```python
from build123d import *

# Parameters (mm, degrees)
SKETCH1_R           = 6.338085432
SKETCH1_W           = 63.5
SKETCH1_H           = 44.45
BOSS_EXTRUDE1_DEPTH = 2.54
BOSS_EXTRUDE2_DEPTH = 12.7
CUT_EXTRUDE1_REACH  = 136.65
SKETCH3_W           = 12.7
SKETCH3_H           = 12.7


with BuildPart() as part:
    # Sketch1 → Boss-Extrude1 (new body)
    with BuildSketch(Plane.XY):
        with BuildLine():
            Line((88.9, 99.06), (88.9, 2.54))
            ThreePointArc((88.9, 2.54), (88.156051224, 0.743948776), (86.36, 0))
            Line((86.36, 0), (2.54, 0))
            ThreePointArc((2.54, 0), (0.743948776, 0.743948776), (0, 2.54))
            Line((0, 2.54), (0, 99.06))
            ThreePointArc((0, 99.06), (0.743948776, 100.856051224), (2.54, 101.6))
            Line((2.54, 101.6), (86.36, 101.6))
            ThreePointArc((86.36, 101.6), (88.156051224, 100.856051224), (88.9, 99.06))
        make_face()
        with Locations((31.75, 25.352341726)):
            Circle(SKETCH1_R, mode=Mode.SUBTRACT)
        with Locations((44.366598021, 38.028512589)):
            Circle(SKETCH1_R, mode=Mode.SUBTRACT)
        with Locations((57.042768884, 25.352341726)):
            Circle(SKETCH1_R, mode=Mode.SUBTRACT)
        with Locations((44.366598021, 12.676170863)):
            Circle(SKETCH1_R, mode=Mode.SUBTRACT)
        with Locations((45.72, 75.565)):
            Rectangle(SKETCH1_W, SKETCH1_H, mode=Mode.SUBTRACT)
    extrude(amount=BOSS_EXTRUDE1_DEPTH)

    # Sketch2 → Boss-Extrude2 (add)
    with BuildSketch(Plane(origin=(0, 0, 0), x_dir=(-1, 0, 0), z_dir=(0, 0, -1))):
        with BuildLine():
            Line((-3.81, 100.33), (-85.09, 100.33))
            ThreePointArc((-85.09, 100.33), (-86.886051224, 99.586051224), (-87.63, 97.79))
            Line((-87.63, 97.79), (-87.63, 3.81))
            ThreePointArc((-87.63, 3.81), (-86.886051224, 2.013948776), (-85.09, 1.27))
            Line((-85.09, 1.27), (-3.81, 1.27))
            ThreePointArc((-3.81, 1.27), (-2.013948776, 2.013948776), (-1.27, 3.81))
            Line((-1.27, 3.81), (-1.27, 97.79))
            ThreePointArc((-1.27, 97.79), (-2.013948776, 99.586051224), (-3.81, 100.33))
        make_face()
        with BuildLine():
            ThreePointArc((-83.82, 99.06), (-85.616051224, 98.316051224), (-86.36, 96.52))
            Line((-86.36, 96.52), (-86.36, 5.08))
            ThreePointArc((-86.36, 5.08), (-85.616051224, 3.283948776), (-83.82, 2.54))
            Line((-83.82, 2.54), (-5.08, 2.54))
            ThreePointArc((-5.08, 2.54), (-3.283948776, 3.283948776), (-2.54, 5.08))
            Line((-2.54, 5.08), (-2.54, 96.52))
            ThreePointArc((-2.54, 96.52), (-3.283948776, 98.316051224), (-5.08, 99.06))
            Line((-5.08, 99.06), (-83.82, 99.06))
        make_face(mode=Mode.SUBTRACT)
    extrude(amount=BOSS_EXTRUDE2_DEPTH)

    # Sketch3 → Cut-Extrude1 (cut, up to next)
    with BuildSketch(Plane.XZ.offset(-1.27), mode=Mode.PRIVATE) as cut_extrude1_sk1:
        with Locations((78.74, -6.35)):
            Rectangle(SKETCH3_W, SKETCH3_H)
    cut_extrude1_tool1 = extrude(cut_extrude1_sk1.sketch, amount=-CUT_EXTRUDE1_REACH, mode=Mode.PRIVATE) & part.part
    add(cut_extrude1_tool1.solids().sort_by_distance((78.74, 1.27, -6.35))[0], mode=Mode.SUBTRACT)


solid = part.part
```
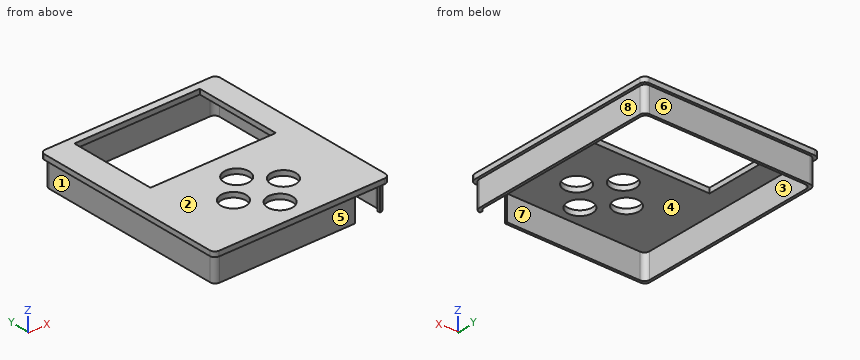
Source: CAD feature listing. Evaluate the final solid. Frame: model axes, mm. Face numbers are marked on the shaded views. A direction names the side the tool comes from. Give positions to 0.01 mm unless a question says otherwise; leave off trailing zeros. Loops run counter-clockwise (first coordinate to the right, second up) from the corner with the lowest first, then second, coordinate; pieces in that order, holes last. Notation, with made-up numbers: (77, 59.25) - (133, 59.25) arc R23 cw to (133, 88.25) - close; hole circle Ø1 at (31.5, 77.25). An arc over 180 degrees is marked (long way). Use CSV: the item, a comma, the result in double quotes. Start each with the question number.
1. Ray query, L1, parallel to Y at x = 31.75, z = 0.6; L2, parallel to Y at x = 24.5, z = -1.25; L3, parallel to X at y = 54.5, z = -4. Return the intervals inside material, ascending.
2. Reachability of the marked faces 5, 6, 7 and 8 from +Z, -Z, +X, -X, +Y, -Y: full face, straight path, thin tool, end or side. Return the list, or none.
3. Section C-C (z = -3.25). Output: boundary loops of the cut face in (x, y), then the cut area to 3 significant figures.
4. Section B-B (y = 65). Output: boundary loops of the cut face in (x, z), then the cut area to 3 significant figures.
5. Pin query (flat end, axial travel): pin 1 (4 mm diameter, centred on y = 61, z = -5.5, fed in from +X); pin 2 (10 mm diameter, centred on x = 57.04, y = 25.35, fed in from +Z); pin 3 (4 mm diameter, centred on x = 64.5, z = -10, fed in from +Y); pin 4 (5 mm diameter, centred on x = 38, z = -5.5, fed in from -Y). Return the tip coordinate at first contact, or that it passes through.
6. Draft query along X for the marked faces 1, 2, 3 and 4. Return one class per face: +X half, -X half, draft (parallel to the pull), parting line (faces both ways), or undercut.
7. Section D-D (y = 22). Output: boundary loops of the cut face in (x, z).
8. Section A-A (x = 31.75). Output: boundary loops of the cut face in (y, z), then the cut area to 3 significant figures.
Response:
1,L1,"0 to 19.01, 31.69 to 53.34, 97.79 to 101.6"
1,L2,"1.27 to 2.54, 99.06 to 100.33"
1,L3,"1.27 to 2.54, 86.36 to 87.63"
2,face 5,"-Z, +X, -X, -Y"
2,face 6,"-Z, +X, -X, +Y"
2,face 7,"-Z"
2,face 8,"-Z, +X, +Y, -Y"
3,outline,"(1.27, 3.81) arc R2.54 ccw to (3.81, 1.27) - (72.39, 1.27) - (72.39, 2.54) - (5.08, 2.54) arc R2.54 cw to (2.54, 5.08) - (2.54, 96.52) arc R2.54 cw to (5.08, 99.06) - (83.82, 99.06) arc R2.54 cw to (86.36, 96.52) - (86.36, 5.08) arc R2.54 cw to (85.09, 2.88) - (85.09, 1.27) arc R2.54 ccw to (87.63, 3.81) - (87.63, 97.79) arc R2.54 ccw to (85.09, 100.33) - (3.81, 100.33) arc R2.54 ccw to (1.27, 97.79) - close"
3,area,"448 mm²"
4,outline,"(0, 0) - (1.27, 0) - (1.27, -12.7) - (2.54, -12.7) - (2.54, 0) - (13.97, 0) - (13.97, 2.54) - (0, 2.54) - close; (77.47, 0) - (86.36, 0) - (86.36, -12.7) - (87.63, -12.7) - (87.63, 0) - (88.9, 0) - (88.9, 2.54) - (77.47, 2.54) - close"
4,area,"96.8 mm²"
5,pin 1,"x = 87.63"
5,pin 2,"through"
5,pin 3,"y = 100.33"
5,pin 4,"y = 1.27"
6,face 1,"-X half"
6,face 2,"draft"
6,face 3,"undercut"
6,face 4,"undercut"
7,outline,"(0, 0) - (1.27, 0) - (1.27, -12.7) - (2.54, -12.7) - (2.54, 0) - (26.37, 0) - (26.37, 2.54) - (0, 2.54) - close; (37.13, 0) - (51.66, 0) - (51.66, 2.54) - (37.13, 2.54) - close; (62.42, 0) - (86.36, 0) - (86.36, -12.7) - (87.63, -12.7) - (87.63, 0) - (88.9, 0) - (88.9, 2.54) - (62.42, 2.54) - close"
8,outline,"(0, 0) - (1.27, 0) - (1.27, -12.7) - (2.54, -12.7) - (2.54, 0) - (19.01, 0) - (19.01, 2.54) - (0, 2.54) - close; (31.69, 0) - (53.34, 0) - (53.34, 2.54) - (31.69, 2.54) - close; (97.79, 0) - (99.06, 0) - (99.06, -12.7) - (100.33, -12.7) - (100.33, 0) - (101.6, 0) - (101.6, 2.54) - (97.79, 2.54) - close"
8,area,"145 mm²"
